Geometry check sheet. Reference: the model listing, model coordinates, mm. A direction names the side the tool comes from. Coordinates: 2 decimals unless noted, no trailing zeros. Order: outer loops, then holes, each group sorted by start corner. A loop starts at its lowest first (then second) coordinate and runs counter-clockwise, first axis right, second up. Notation, with made-up numbers: M -9,-25.75 L 11,-25.75 A26 cw 11,2.25 Z; hole C 72.25,-12 d8. An arc over 180 degrees is marked long. One line per item, written item: value. Start each with the question number.
1) Thickness scan on L1, parallel to Y at x = 45.5, z = 7; L2, parallel to X at y = -23.25, z = 1.3; L3, parallel to Z at x = 48.5, y = -8. Record the ranges inside material, lowest first. Write a range as from..to.
2) Sectioned sample at C-C, the plane z = 8. Enter the section's corners in (x, y).
3) Draft check along X on faces 4 (the flat face through (0, -19, 5)), 5 (the flat face through (45, -38, 5)), 6 (the cylindrical face through (52.26, -15.21, 0.99)), 7 (the cylindrical face through (45.5, -9, 1)). Enter one of: pulls with the +X half, pulls with the -X half, needs draft (parallel to the pull), parting line crosses it, or undercut.
4) Sectioned sample at D-D, the plane y = -29.5. Enter the section's corners in (x, z), then the cut area to 3 significant figures.
5) Sectioned sample at A-A, the plane x = 45.5. Enter the section's corners in (y, z), then the cut area to 4 significant figures.
6) Go/stop test with flat-tipped pins: P1, Ø7, axis at x = 48.5, y = -22.5, coming from the +Z side; P2, Ø2.5, axis at x = 45.5, y = -10.5, coming from the +Z side. Record where each tip stops, or that it passes through.
7) Sectioned sample at B-B, the plane y = -19. Enter the section's corners in (x, z), then the cut area to 3 significant figures.
8) Access from +Z, -Z, +X, -X, +Y, -Y to the whole of each face (thin tool, end or side, straight path). Record for faces 1 (the flat face through (44.9, -31.4, 10)), 2 (the cylindrical face through (38.84, -15.04, 0.99)), 3 (the cylindrical face through (36.656, -10.89, 6.056)).
```python
from build123d import *

# Parameters (mm, degrees)
ESQUISSE1_W      = 91
ESQUISSE1_H      = 38
EXTRUSION1_DEPTH = 10
ESQUISSE3_R      = 12
EXTRUSION3_DEPTH = 8


with BuildPart() as part:
    # Esquisse1 → Extrusion1 (new body)
    with BuildSketch(Plane.XY):
        with Locations((45.5, -19)):
            Rectangle(ESQUISSE1_W, ESQUISSE1_H)
        with BuildLine():
            ThreePointArc((44.263573917, -11.349264706), (38.788303121, -15.125), (38.256055836, -21.754591249))
            ThreePointArc((38.256055836, -21.754591249), (36.839745962, -24), (39.492481919, -23.896144045))
            ThreePointArc((39.492481919, -23.896144045), (45.5, -26.75), (51.507518081, -23.896144045))
            ThreePointArc((51.507518081, -23.896144045), (54.160254038, -24), (52.743944164, -21.754591249))
            ThreePointArc((52.743944164, -21.754591249), (52.211696879, -15.125), (46.736426083, -11.349264706))
            ThreePointArc((46.736426083, -11.349264706), (45.5, -9), (44.263573917, -11.349264706))
        make_face(mode=Mode.SUBTRACT)
    extrude(amount=EXTRUSION1_DEPTH)

    # Esquisse3 → Extrusion3 (cut)
    with BuildSketch(Plane.XY.offset(10)):
        with Locations((45.5, -19)):
            Circle(ESQUISSE3_R)
    extrude(amount=-EXTRUSION3_DEPTH, mode=Mode.SUBTRACT)


solid = part.part
```
Final values:
1. L1: y = -38..-31, -7..0
1. L2: x = 0..36.64, 54.36..91
1. L3: z = 0..2
2. outline: M 0,-38 L 91,-38 L 91,0 L 0,0 Z; hole C 45.5,-19 d24
3. face 4: pulls with the -X half
3. face 5: needs draft
3. face 6: undercut
3. face 7: undercut
4. outline: M 0,0 L 91,0 L 91,10 L 51.31,10 L 51.31,2 L 39.69,2 L 39.69,10 L 0,10 Z
4. area: 817 mm^2
5. outline: M -38,0 L -26.75,0 L -26.75,2 L -31,2 L -31,10 L -38,10 Z; M -9,0 L 0,0 L 0,10 L -7,10 L -7,2 L -9,2 Z
5. area: 152.5 mm^2
6. P1: stops at z = 2
6. P2: passes through
7. outline: M 0,0 L 37.75,0 L 37.75,2 L 33.5,2 L 33.5,10 L 0,10 Z; M 53.25,0 L 91,0 L 91,10 L 57.5,10 L 57.5,2 L 53.25,2 Z
7. area: 687 mm^2
8. face 1: +Z, +X, -X, +Y, -Y
8. face 2: +Z, -Z
8. face 3: +Z
